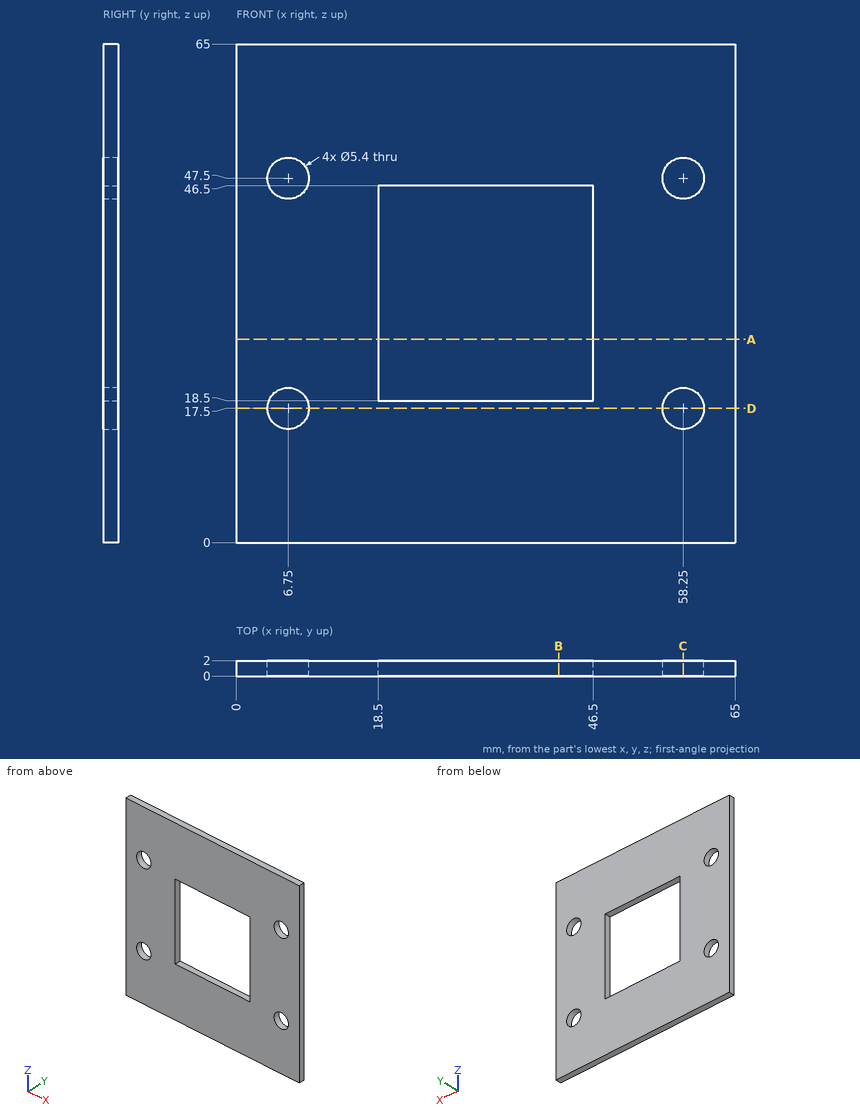
Design review of the part shown in the three views and the two pictorial views. Dimensions are in mm from the part's minimum x, y and z. Round coordinates to 2 decimals unless told otherwise and drop trailing zeros. Loops run counter-clockwise (first coordinate to the right, second up) from the corner with the lowest first, then second, coordinate; pieces in that order, holes last. Notation, with made-up numbers: (29.25, 1.25) -> (50.25, 1.25) arc R22 ccw to (50.25, 25.25) -> close; hole circle Ø6 at (-6.5, 2). An arc over 180 degrees is marked (long way). Return JSON: item names as keys, results as strings.
(1) Add section B-B on x = 42. Write out the cut boundary in (y, z).
Solved:
{"outline": "(0, 0) -> (2, 0) -> (2, 18.5) -> (0, 18.5) -> close; (0, 46.5) -> (2, 46.5) -> (2, 65) -> (0, 65) -> close"}
(2) Add section A-A on z = 26.5. Write out the cut boundary in (x, y), plus the area to 3 significant figures.
Solved:
{"outline": "(0, 0) -> (18.5, 0) -> (18.5, 2) -> (0, 2) -> close; (46.5, 0) -> (65, 0) -> (65, 2) -> (46.5, 2) -> close", "area": "74.0 mm2"}
(3) For line 1 (X direction, y = 0.5, z = 17.5); line 2 (Z direction, x = 27.5, y = 0.35); line 3 (Z direction, x = 58.5, y = 1.1), list the stretches that pass through material, from the lowest coordinate up.
Solved:
{"line 1": "0 to 4.05, 9.45 to 55.55, 60.95 to 65", "line 2": "0 to 18.5, 46.5 to 65", "line 3": "0 to 14.81, 20.19 to 44.81, 50.19 to 65"}
(4) Add section D-D on z = 17.5. Write out the cut boundary in (x, y), plus the area to 3 significant figures.
Solved:
{"outline": "(0, 0) -> (4.05, 0) -> (4.05, 2) -> (0, 2) -> close; (9.45, 0) -> (55.55, 0) -> (55.55, 2) -> (9.45, 2) -> close; (60.95, 0) -> (65, 0) -> (65, 2) -> (60.95, 2) -> close", "area": "108 mm2"}
(5) For pin 1 (3 mm diameter, centred on x = 58.25, z = 47.5, fed in from -Y), flat-tipped, find the tip position at first contact; note if it passes through.
Solved:
{"pin 1": "through"}
(6) Add section C-C on x = 58.25. Write out the cut boundary in (y, z), plus the area to 3 significant figures.
Solved:
{"outline": "(0, 0) -> (2, 0) -> (2, 14.8) -> (0, 14.8) -> close; (0, 20.2) -> (2, 20.2) -> (2, 44.8) -> (0, 44.8) -> close; (0, 50.2) -> (2, 50.2) -> (2, 65) -> (0, 65) -> close", "area": "108 mm2"}
